For this review, take the finished solid that the model builds, in its own axes (mm). Face numbers are marked on the shaded views. A direction names the side the tool comes from. Give positions to 0.01 mm unless a question says otherwise; leave off trailing zeros. Loops run counter-clockwise (first coordinate to the right, second up) from the corner with the lowest first, then second, coordinate; pieces in that order, holes last. Notation, with made-up numbers: (13.25, 30.25) -> (44.25, 30.25) arc R16 ccw to (44.25, 34.25) -> close; hole circle Ø1 at (87.25, -23). An arc over 180 degrees is marked (long way). Answer as CSV lines item,"result". Start each with the question number.
Item 1: Machinability: for the marked faces 5 and 6, which of the approach directions +Z, -Z, +X, -X, +Y, -Y give a long, thin tool a straight path to every point of the face, cutting with its end or side? Answer none if there is none.
Item 2: Clearance check with a flat-ended pin moving along its axis: P1, Ø10, axis at x = 11, z = 6, coming from the +Y side. State where the tip first meets the part, or that it passes through.
Item 3: Add section C-C on x = 15.5. State the section outline as (y, z) points, plus the area to 3 significant figures.
Item 4: For L1, parallel to X at y = 13.5, z = 9.5; L2, parallel to Y at x = 11, z = 19.25; L3, parallel to Y at x = 14.5, z = 20, list the stretches that pass through material, from the lowest coordinate up. Write a range as from..to.
Item 5: Add section A-A on z = 11. State the section outline as (x, y) points.
Item 6: The part is to be moulded in two halves that separate along Y. For the marked faces 1, 2, 3 and 4, say which applies: +Y half, -Y half, draft (parallel to the pull), parting line (faces both ways), or undercut.
Item 7: Add section D-D on y = 28. State the section outline as (x, z) points.
Item 8: Add section B-B on y = 21. State the section outline as (x, z) points, plus the area to 3 significant figures.
```python
from build123d import *

# Parameters (mm, degrees)
SZKIC1_W                    = 43
SZKIC1_H                    = 45
DODANIE_WYCI_GNI_CIE1_DEPTH = 22
SZKIC3_W                    = 28
SZKIC3_H                    = 35
WYTNIJ_WYCI_GNI_CIE1_DEPTH  = 63
SZKIC4_R                    = 7.5
WYTNIJ_WYCI_GNI_CIE2_DEPTH  = 63
ZAOKR_GLENIE1_R             = 10
ZAOKR_GLENIE2_R             = 2
ZAOKR_GLENIE3_R             = 5


with BuildPart() as part:
    # Szkic1 → Dodanie-wyciągnięcie1 (new body)
    with BuildSketch(Plane.XY):
        with Locations((0, 22.5)):
            Rectangle(SZKIC1_W, SZKIC1_H)
    extrude(amount=DODANIE_WYCI_GNI_CIE1_DEPTH)

    # Szkic3 → Wytnij-wyciągnięcie1 (cut)
    with BuildSketch(Plane.XY):
        with Locations((0, 27.5)):
            Rectangle(SZKIC3_W, SZKIC3_H)
    extrude(amount=WYTNIJ_WYCI_GNI_CIE1_DEPTH, mode=Mode.SUBTRACT)

    # Szkic4 → Wytnij-wyciągnięcie2 (cut)
    with BuildSketch(Plane(origin=(21.5, 0, 0), x_dir=(0, 0, -1), z_dir=(1, 0, 0))):
        with Locations((-11, 33.5)):
            Circle(SZKIC4_R)
    extrude(amount=-WYTNIJ_WYCI_GNI_CIE2_DEPTH, mode=Mode.SUBTRACT)

    # Zaokrąglenie1
    zaokr_glenie1_edges = [part.edges().sort_by_distance(p)[0] for p in [
        (-17.75, 45, 0),
        (-17.75, 45, 22),
        (17.75, 45, 22),
        (17.75, 45, 0),
    ]]
    fillet(zaokr_glenie1_edges, radius=ZAOKR_GLENIE1_R)

    # Zaokrąglenie2
    zaokr_glenie2_edges = [part.edges().sort_by_distance(p)[0] for p in [
        (14, 10, 11),
        (-14, 10, 11),
    ]]
    fillet(zaokr_glenie2_edges, radius=ZAOKR_GLENIE2_R)

    # Zaokrąglenie3
    zaokr_glenie3_edges = [part.edges().sort_by_distance(p)[0] for p in [
        (21.5, 0, 11),
        (-21.5, 0, 11),
    ]]
    fillet(zaokr_glenie3_edges, radius=ZAOKR_GLENIE3_R)


solid = part.part
```
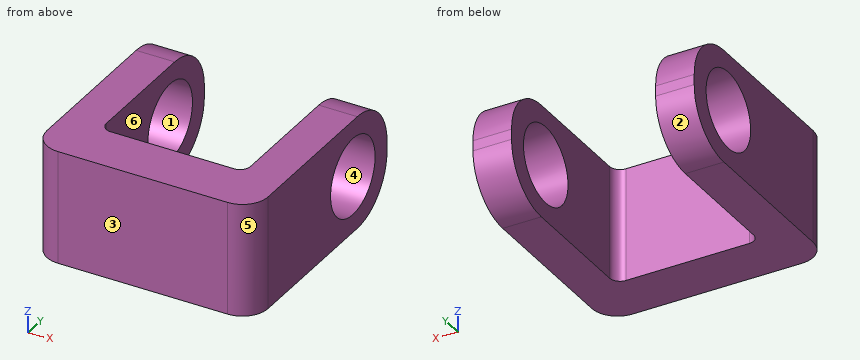
Computed values:
1,face 5,"+Z, -Z, +X, -Y"
1,face 6,"+Z, -Z, +Y"
2,P1,"y = 45"
3,outline,"(0, 0) -> (35, 0) arc R10 ccw to (45, 10) -> (45, 12) arc R10 ccw to (35, 22) -> (0, 22) -> close; hole circle Ø15 at (33.5, 11)"
3,area,"770 mm²"
4,L1,"-21.5..-14, 14..21.5"
4,L2,"0..10"
4,L3,"0..41"
5,outline,"(-21.5, 5) arc R5 ccw to (-16.5, 0) -> (16.5, 0) arc R5 ccw to (21.5, 5) -> (21.5, 26) -> (14, 26) -> (14, 12) arc R2 cw to (12, 10) -> (-12, 10) arc R2 cw to (-14, 12) -> (-14, 26) -> (-21.5, 26) -> close; (-21.5, 41) -> (-14, 41) -> (-14, 45) -> (-21.5, 45) -> close; (14, 41) -> (21.5, 41) -> (21.5, 45) -> (14, 45) -> close"
6,face 1,"undercut"
6,face 2,"+Y half"
6,face 3,"-Y half"
6,face 4,"undercut"
7,outline,"(-21.5, 0) -> (-14, 0) -> (-14, 5.9) -> (-21.5, 5.9) -> close; (-21.5, 16.1) -> (-14, 16.1) -> (-14, 22) -> (-21.5, 22) -> close; (14, 0) -> (21.5, 0) -> (21.5, 5.9) -> (14, 5.9) -> close; (14, 16.1) -> (21.5, 16.1) -> (21.5, 22) -> (14, 22) -> close"
8,outline,"(-21.5, 0) -> (-14, 0) -> (-14, 22) -> (-21.5, 22) -> close; (14, 0) -> (21.5, 0) -> (21.5, 22) -> (14, 22) -> close"
8,area,"330 mm²"
